CAD build for the part. Positions are in the model's coordinates, mm. Face numbers are marked on the shaded views. A direction names the side the tool comes from. Round coordinates to 2 decimals unless told otherwise and drop trailing zeros. Loops run counter-clockwise (first coordinate to the right, second up) from the corner with the lowest first, then second, coordinate; pieces in that order, holes last. Notation, with made-up numbers: M -6.75,33 L 20.25,33 A25 cw 20.25,60 Z; hole C 63.25,10 d1. An arc over 180 degrees is marked long. Use a Markdown table: item, result. Add a question column.
(1) Which spindle directions (+Z, -Z, +X, -X, +Y, -Y) get a long thin tool onto all of the face, cutting with end or side? Do the marked faces 1 and 2. Say none if no direction does.
(2) Flat gauge pins, fed straight in: P1, Ø10, axis at x = 395, z = -40, coming from the +Y side; P2, Ø1.5, axis at x = 122, y = 20, coming from the +Z side. Where does each tip first touch, or does it go through?
(3) Wall check: L1, parallel to Y at x = 361, z = -54; L2, parallel to Z at x = 404, y = 15. Give the ranges that are in metal, low to high.
(4) Band-saw the part on C-C, the plane y = 77. Write the cut outline in (x, z).
(5) Band-saw the part on A-A, the plane x = 283. Write the cut outline in (y, z).
(6) Band-saw the part on B-B, the plane z = -19. Write the cut outline in (x, y), and give its area (3 significant figures).
from build123d import *

# Parameters (mm, degrees)
SKETCH1_W                    = 457.2
SKETCH1_H                    = 57.15
BASE_FLANGE1_DEPTH           = 0.15875
EDGE_FLANGE1_STRIP_W         = 2.1082
EDGE_FLANGE1_STRIP_H         = 0.15875
EDGE_FLANGE1_STRIP_CUT_DEPTH = 457.2
EDGE_FLANGE1_DEPTH           = 457.2
CUT_EXTRUDE1_DEPTH           = 488.3392299
F_1_4_CLEARANCE_HOLE2_D      = 6.7564
F_1_4_CLEARANCE_HOLE2_DEPTH  = 25.4
F_1_4_CLEARANCE_HOLE2_TIP    = 2.029827343


# Sheet-metal steps are written as plain solids
with BuildPart() as part:
    # Sketch1 → Base-Flange1 (new body)
    with BuildSketch(Plane(origin=(0, 0, 0), x_dir=(1, 0, 0), z_dir=(0, 1, 0))):
        with Locations((228.6, 28.575)):
            Rectangle(SKETCH1_W, SKETCH1_H)
    extrude(amount=-BASE_FLANGE1_DEPTH)

    # Edge-Flange1 strip (across the edge) → Edge-Flange1 strip cut (cut)
    with BuildSketch(Plane(origin=(457.2, 0, -57.15), x_dir=(0, 0, 1), z_dir=(-1, 0, 0))):
        with Locations((-0.15875, -0.079375)):
            Rectangle(EDGE_FLANGE1_STRIP_W, EDGE_FLANGE1_STRIP_H)
    extrude(amount=EDGE_FLANGE1_STRIP_CUT_DEPTH, mode=Mode.SUBTRACT)

    # Edge-Flange1 section (across the edge) → Edge-Flange1 (add)
    with BuildSketch(Plane(origin=(457.2, 0, -57.15), x_dir=(0, 0, 1), z_dir=(-1, 0, 0))):
        with BuildLine():
            Line((0, 0.7366), (0, 158.75))
            Line((0, 158.75), (0.15875, 158.75))
            Line((0.15875, 158.75), (0.15875, 0.7366))
            ThreePointArc((0.15875, 0.7366), (0.374495145, 0.215745145), (0.89535, 0))
            Line((0.89535, 0), (0.89535, -0.15875))
            ThreePointArc((0.89535, -0.15875), (0.262241943, 0.103491943), (0, 0.7366))
        make_face()
    extrude(amount=EDGE_FLANGE1_DEPTH)

    # Sketch9 → Cut-Extrude1 (cut, through all)
    with BuildSketch(Plane(origin=(0, 0, -57.15), x_dir=(-1, 0, 0), z_dir=(0, 0, -1))):
        with BuildLine():
            Line((-446.278, 152.4), (-446.278, 158.75))
            Line((-446.278, 158.75), (-452.882, 158.75))
            Line((-452.882, 158.75), (-452.882, 152.4))
            ThreePointArc((-452.882, 152.4), (-449.58, 149.098), (-446.278, 152.4))
        make_face()
        with BuildLine():
            Line((-10.922, 152.4), (-10.922, 158.75))
            Line((-10.922, 158.75), (-4.318, 158.75))
            Line((-4.318, 158.75), (-4.318, 152.4))
            ThreePointArc((-4.318, 152.4), (-7.62, 149.098), (-10.922, 152.4))
        make_face()
    extrude(amount=-CUT_EXTRUDE1_DEPTH, mode=Mode.SUBTRACT)

    # 1/4 Clearance Hole2
    with Locations(Plane(origin=(10.16, -0.15875, -10.16), x_dir=(0, 0, -1), z_dir=(0, -1, 0))):
        with Locations((0, 0), (0, 436.88)):
            Hole(F_1_4_CLEARANCE_HOLE2_D / 2, depth=F_1_4_CLEARANCE_HOLE2_DEPTH)
            with Locations((0, 0, -(F_1_4_CLEARANCE_HOLE2_DEPTH + F_1_4_CLEARANCE_HOLE2_TIP / 2))):  # 118° drill point
                Cone(0, F_1_4_CLEARANCE_HOLE2_D / 2, F_1_4_CLEARANCE_HOLE2_TIP, mode=Mode.SUBTRACT)


solid = part.part
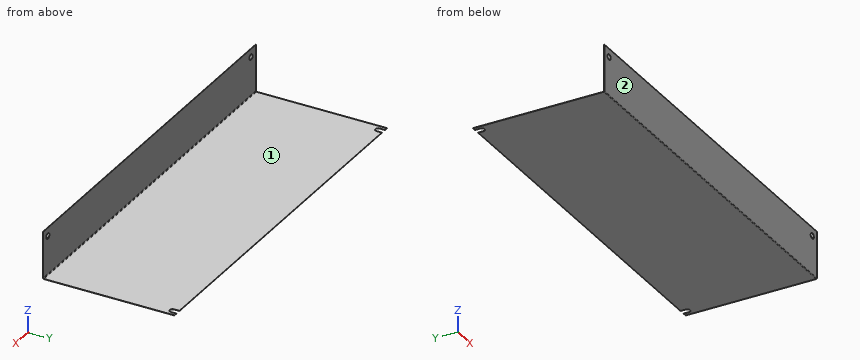
Return value:
| question | item | result |
|---|---|---|
| 1 | face 1 | +Z, +X, -X, +Y |
| 1 | face 2 | +Z, -Z, +X, -X, -Y |
| 2 | P1 | y = 0 |
| 2 | P2 | z = -56.99 |
| 3 | L1 | -0.16 to 0 |
| 3 | L2 | -57.15 to -56.99 |
| 4 | outline | M 0,-57.15 L 457.2,-57.15 L 457.2,-56.99 L 0,-56.99 Z |
| 5 | outline | M -0.16,-56.25 A0.9 ccw 0.74,-57.15 L 158.75,-57.15 L 158.75,-56.99 L 0.74,-56.99 A0.74 cw 0,-56.25 L 0,0 L -0.16,0 Z |
| 6 | outline | M 0,-0.16 L 457.2,-0.16 L 457.2,0 L 0,0 Z |
| 6 | area | 72.6 mm^2 |
